Study the drawing (mm; zero at the part's minimum x, y, z) and answer. A direction names the side the tool comes from. Give positions to 0.01 mm unless a question says otherwise; leave off trailing zeros. Write each loop counter-clockwise with the first axis right and the second up, starting at its lowest first coordinate (ties: lowest second). Pieces come first, ordered by that corner, then holes. Notation, with made-up numbers: M 74,37.5 L 84,37.5 A14 ccw 84,62.5 Z; hole C 38,-20 d3. An arc over 180 degrees is marked long. Use a Markdown table: item, result. Add a question column.
Item 1: A cutting plane is placed at B-B on x = 3.5. Determine the outline of the cut face in (y, z) (1 decimal).
Item 2: A cutting plane is placed at D-D on z = 15. Determine the outline of the cut face in (x, y).
Item 3: A cutting plane is placed at A-A on y = 4. Determine the outline of the cut face in (x, z) (1 decimal), then the cut area to 3 significant figures.
Item 4: The mould has two halves that part along Y. Classify the marked faces 1 and 2: pulls with the +Y half, pulls with the -Y half, needs draft (parallel to the pull), parting line crosses it, or undercut.
Item 5: Consider probe 1 along Y at (x, z) = (7.75, 7); probe 2 along Z at (x, y) = (7, 13.5); probe 3 along Z at (x, y) = (13.5, 2.5) (1 decimal). Determine where each line is inside the solid, lowest interval first. Write a range as [from, to].
Item 6: Given P1, Ø1, axis at x = 3.5, y = 2.5, coming from the -Z side (1 decimal); P2, Ø5, axis at x = 5.5, z = 13, coming from the +Y side; P3, Ø5, axis at x = 9, z = 13.5, coming from the -Y side (1 decimal); P4, Ø8, axis at y = 10.5, z = 21, coming from the -X side, each flat-ended and moving along its own axis, determine where each tip first touches the part or whether it passes through.
Item 7: For the marked faces 3 and 4, determine the directions among +Z, -Z, +X, -X, +Y, -Y from which every point of the face is accessible in a straight line to the end or side of a thin tool.
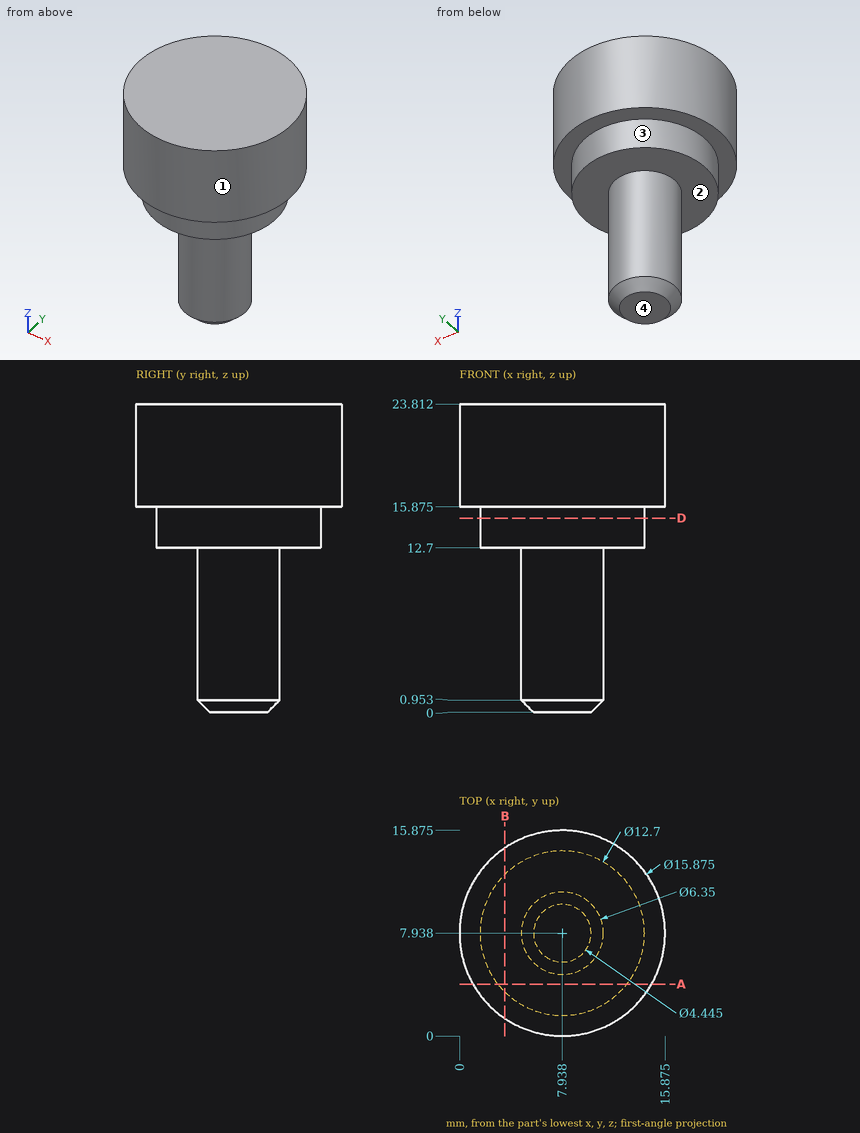
Filled in:
| question | item | result |
|---|---|---|
| 1 | outline | M 1.4,15.9 L 3.4,15.9 L 3.4,12.7 L 12.5,12.7 L 12.5,15.9 L 14.5,15.9 L 14.5,23.8 L 1.4,23.8 Z |
| 2 | outline | C 7.94,7.94 d12.7 |
| 3 | outline | M 1,15.9 L 3,15.9 L 3,12.7 L 12.9,12.7 L 12.9,15.9 L 14.8,15.9 L 14.8,23.8 L 1,23.8 Z |
| 3 | area | 141 mm² |
| 4 | face 1 | parting line crosses it |
| 4 | face 2 | needs draft |
| 5 | probe 1 | [4.77, 11.11] |
| 5 | probe 2 | [12.7, 23.81] |
| 5 | probe 3 | [15.9, 23.8] |
| 6 | P1 | z = 15.9 |
| 6 | P2 | y = 14.29 |
| 6 | P3 | y = 0 |
| 6 | P4 | x = 0 |
| 7 | face 3 | -Z |
| 7 | face 4 | -Z, +X, -X, +Y, -Y |
